Autodesk Inventor part; units mm, degrees
ref_plane "YZ Plane" through (0, 0, 0) normal (1, 0, 0) x (0, 1, 0)
ref_plane "XZ Plane" through (0, 0, 0) normal (0, 1, 0) x (-1, 0, 0)
ref_plane "XY Plane" through (0, 0, 0) normal (0, 0, 1) x (1, 0, 0)
sketch "Sketch1" plane through (0, 0, 0) normal (1, 0, 0) x (0, 1, 0)
  line L0 (-63.921, 100) -> (63.921, 100)
  line L1 (63.921, 100) -> (63.921, -100)
  line L2 (63.921, -100) -> (-63.921, -100)
  line L3 (-63.921, -100) -> (-63.921, 100)
  line L4 (-63.921, 100) -> (63.921, -100) construction
  line L5 (63.921, 100) -> (-63.921, -100) construction
  line L6 (63.921, 50) -> (-36.079, 50)
  line L7 (-36.079, 50) -> (-36.079, -50)
  line L8 (-36.079, -50) -> (63.921, -50)
  line L9 (63.921, -50) -> (63.921, 50)
  point P0 (0, 0)
  point P1 (63.921, -50)
  dimension "d0" = 200
  dimension "d1" = 127.842
  dimension "d2" = 100
  dimension "d3" = 100
  dimension "d4" = 50
extrude "Extrusion1" add sketch "Sketch1" along normal blind 3 contours L0 L1 L6 L7 L8 L2 L3
equation "\"d3\" = d2"
properties part number "WI-CoverRS3"
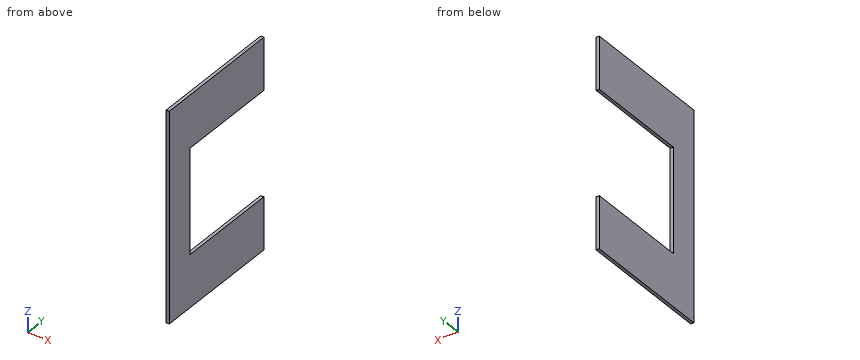
Geometry check sheet. Reference: the model listing, model coordinates, mm. Round coordinates to 2 decimals unless told otherwise and drop trailing zeros. Loops run counter-clockwise (first coordinate to the right, second up) from the corner with the lowest first, then second, coordinate; pieces in that order, holes last.
Item 1: Cross-section at B-B on x = 2.3. Record the boundary of the cut face in (y, z).
Item 2: Thickness scan on line 1 (Z direction, x = 0.65, y = 40.5); line 2 (Y direction, x = 2.85, z = 8). Record the ranges inside material, lowest first.
Item 3: Cross-section at C-C on z = 4. Record the boundary of the cut face in (x, y).
Item 4: Cross-section at A-A on y = 15.5. Record the boundary of the cut face in (x, z).
Answer sheet:
1. outline: (-63.92, -100) - (63.92, -100) - (63.92, -50) - (-36.08, -50) - (-36.08, 50) - (63.92, 50) - (63.92, 100) - (-63.92, 100) - close
2. line 1: z = -100 to -50, 50 to 100
2. line 2: y = -63.92 to -36.08
3. outline: (0, -63.92) - (3, -63.92) - (3, -36.08) - (0, -36.08) - close
4. outline: (0, -100) - (3, -100) - (3, -50) - (0, -50) - close; (0, 50) - (3, 50) - (3, 100) - (0, 100) - close
